Could you check a few things on this drawing? It's one solid part, dimensions in mm from its lowest x, y, z. Give positions to 0.01 mm unless a question says otherwise; leave off trailing zeros. Write each loop counter-clockwise with the first axis right and the second up, starting at its lowest first coordinate (ties: lowest second). Pieces come first, ordered by that corner, then holes. Notation, with made-up numbers: M 3,-28 L 54,-28 A12 ccw 54,-20 Z; hole C -30,33 d11. An arc over 180 degrees is marked long. Write each question's results on one line, items separated by ' | '.
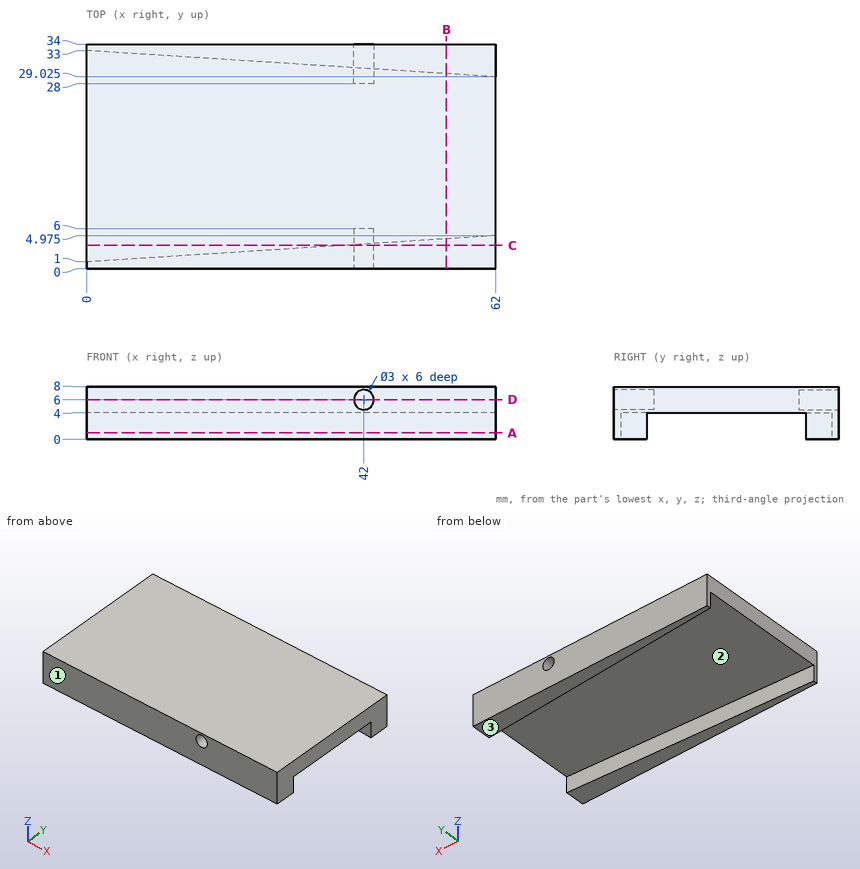
Item 1: I'm going to push flat-ended pins straight in: pin 1 (2.5 mm diameter, centred on x = 42, z = 6, fed in from -Y); pin 2 (3.5 mm diameter, centred on x = 42, z = 6, fed in from -Y); pin 3 (8 mm diameter, centred on x = 28.5, y = 19, fed in from -Z). Where does each tip first touch, or does it pass through?
Geometry says:
pin 1: stops at y = 6 | pin 2: stops at y = 0 | pin 3: stops at z = 4
Item 2: I want a section at A-A, the plane z = 1. Please give me the cut outline in (x, y) (1 decimal).
Geometry says:
outline: M 0,0 L 62,0 L 62,5 L 0,1 Z; M 0,33 L 62,29 L 62,34 L 0,34 Z
Item 3: Thinking about a two-plate mould opening in Y: for the marked faces 1, 2 and 3, which applies, +Y half, -Y half, draft (parallel to the pull), parting line (faces both ways), or undercut?
Geometry says:
face 1: -Y half | face 2: undercut | face 3: draft
Item 4: I want a section at D-D, the plane z = 6. Please give me the cut outline in (x, y), and give its area (3 significant figures).
Geometry says:
outline: M 0,0 L 40.5,0 L 40.5,6 L 43.5,6 L 43.5,0 L 62,0 L 62,34 L 43.5,34 L 43.5,28 L 40.5,28 L 40.5,34 L 0,34 Z | area: 2,070 mm2
Item 5: If I drill on line 1 (Z direction, x = 42, y = 4); line 2 (Z direction, x = 42, y = 3); line 3 (Z direction, x = 49, y = 18), over which ranges is the centre line in solid material (lowest first)? Write a range as from..to.
Geometry says:
line 1: z = 4..4.5, 7.5..8 | line 2: z = 0..4.5, 7.5..8 | line 3: z = 4..8
Item 6: I want a section at C-C, the plane y = 3.5. Please give me the cut outline in (x, z), and give its area (3 significant figures).
Geometry says:
outline: M 0,4 L 38.99,4 L 38.99,0 L 62,0 L 62,8 L 0,8 Z; hole C 42,6 d3 | area: 333 mm2
Item 7: I want a section at B-B, the plane x = 54.5. Please give me the cut outline in (y, z) (1 decimal).
Geometry says:
outline: M 0,0 L 4.5,0 L 4.5,4 L 29.5,4 L 29.5,0 L 34,0 L 34,8 L 0,8 Z
